Check sheet for the drawn part. Datum: minimum x, y, z corner. Units: mm. Coordinates: 2 decimals unless noted, no trailing zeros. Loops run counter-clockwise (first coordinate to the right, second up) from the corner with the lowest first, then second, coordinate; pieces in that order, holes last.
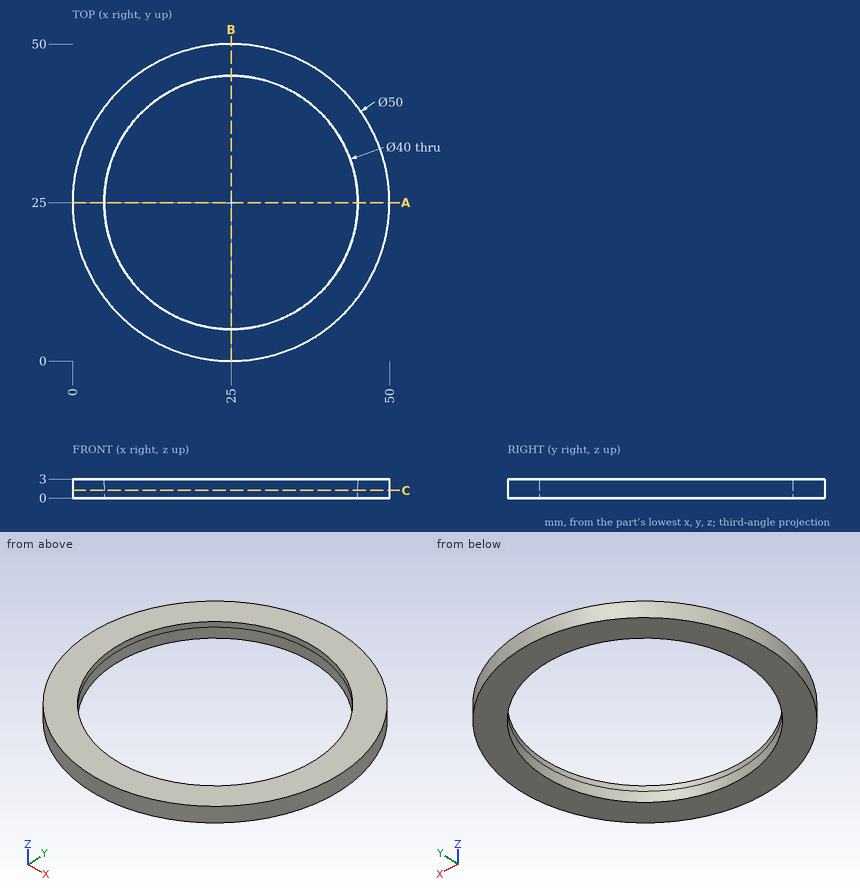
1) Section check C-C on z = 1.2. Enter the section's corners in (x, y).
Answer sheet:
outline: circle Ø50 at (25, 25); hole circle Ø40 at (25, 25)
2) Scan lines: line 1 (Y direction, x = 25, z = 1.4); line 2 (X direction, y = 41.5, z = 0.45); line 3 (Y direction, x = 11, z = 0.4). Record each from-to range of solid material in increasing order.
Answer sheet:
line 1: y = 0 to 5, 45 to 50
line 2: x = 6.22 to 13.7, 36.3 to 43.78
line 3: y = 4.29 to 10.72, 39.28 to 45.71
3) Depth check by flat-ended pin: pin 1 (1.5 mm diameter, centred on x = 8.5, z = 1, fed in from -Y); pin 2 (1 mm diameter, centred on y = 10.5, z = 2.5, fed in from -X); pin 3 (1 mm diameter, centred on y = 28.5, z = 0.5, fed in from -X). Enter the tip coordinate at first touch or a pass-through.
Answer sheet:
pin 1: stops at y = 5.59
pin 2: stops at x = 4.29
pin 3: stops at x = 0.18
4) Section check A-A on y = 25. Enter the section's corners in (x, z).
Answer sheet:
outline: (0, 0) - (5, 0) - (5, 3) - (0, 3) - close; (45, 0) - (50, 0) - (50, 3) - (45, 3) - close
